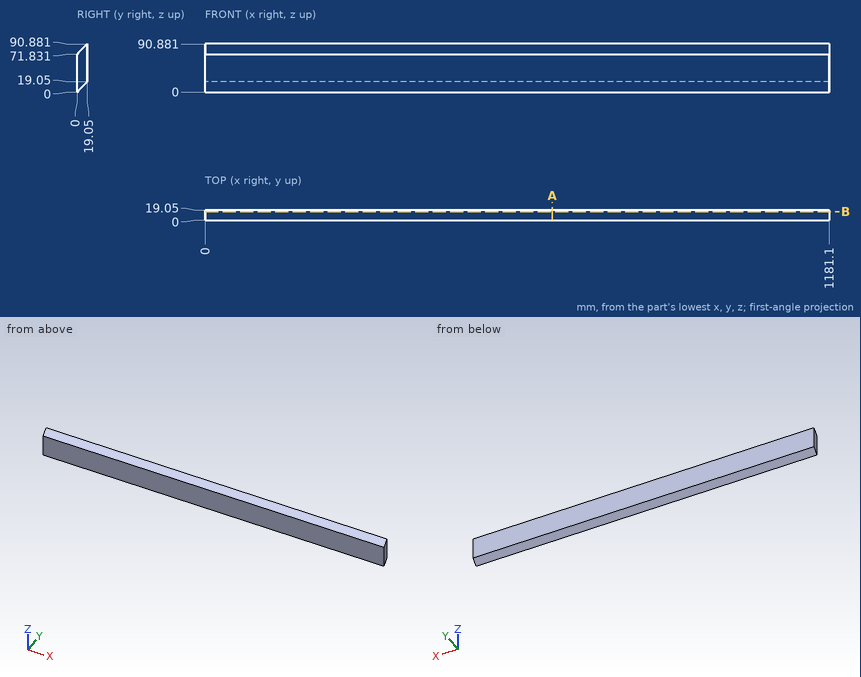
The figure shows three views and two pictorial views of one solid part (mm, origin at its lowest corner). Answer the questions. Coordinates: 2 decimals unless noted, no trailing zeros. Write each loop counter-clockwise with the first axis right and the second up, starting at its lowest first coordinate (ties: lowest second). Pieces come first, ordered by that corner, then holes. Notation, with made-up numbers: (82, 54.25) -> (118, 54.25) arc R17 cw to (118, 76.25) -> close; hole circle Ø11 at (-16, -13.5). An arc over 180 degrees is marked (long way). Return JSON: item names as keys, results as strings.
(1) Consider line 1 along Z through (x, y) = (521, 12); line 2 along Z through (x, y) = (562, 8.75); line 3 along Y through (x, z) = (1003.5, 6.5). Determine where each line is inside the solid, lowest interval first. Write a range as from..to.
Answers below:
{"line 1": "12..83.83", "line 2": "8.75..80.58", "line 3": "0..6.5"}
(2) The part is cut by section A-A on x = 657.5. Give the vertices of the cut face in (y, z).
Answers below:
{"outline": "(0, 0) -> (19.05, 19.05) -> (19.05, 90.88) -> (0, 71.83) -> close"}
(3) Each of these flat-tipped pins is pushed along its axis until it touches: P1, Ø10, axis at y = 14.5, z = 51.5, coming from the -X side; P2, Ø3, axis at x = 615, y = 14, coming from the -Z side. Where does it stop, or does it pass through?
Answers below:
{"P1": "x = 0", "P2": "z = 12.5"}
(4) The part is cut by section B-B on y = 15.75. Give the vertices of the cut face in (x, z).
Answers below:
{"outline": "(0, 15.75) -> (1181.1, 15.75) -> (1181.1, 87.58) -> (0, 87.58) -> close"}
